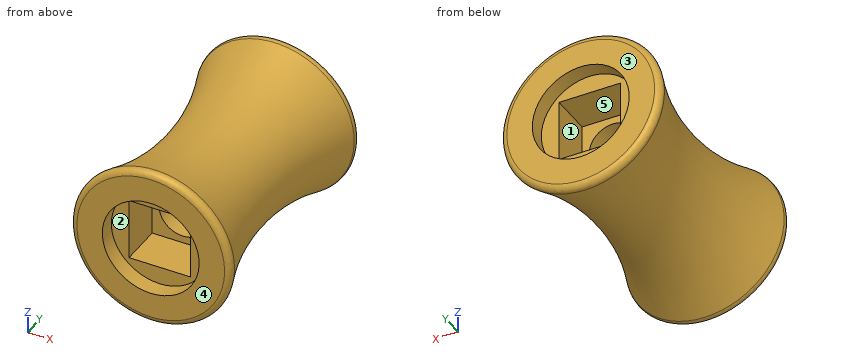
from build123d import *

# Parameters (mm, degrees)
SKETCH2_W           = 6.604
SKETCH2_H           = 6.604
CUT_EXTRUDE1_DEPTH  = 29.341210278
SKETCH3_R           = 5.207
CUT_EXTRUDE2_DEPTH  = 1.778
FILLET1_R           = 0.635
SKETCH4_W           = 6.604
SKETCH4_H           = 6.604
SKETCH4_R           = 2.54
BOSS_EXTRUDE1_DEPTH = 6.35


with BuildPart() as part:
    # Sketch1 → Revolve1 (revolve)
    with BuildSketch(Plane(origin=(0, 0, 0), x_dir=(0, 0, -1), z_dir=(1, 0, 0))):
        with BuildLine():
            Line((2.54, 0), (2.54, 25.4))
            Line((2.54, 25.4), (8.89, 25.4))
            ThreePointArc((8.89, 25.4), (6.239355663, 12.7), (8.89, 0))
            Line((8.89, 0), (2.54, 0))
        make_face()
    revolve(axis=Axis((0, 0, 0), (0, 1, 0)))

    # Sketch2 → Cut-Extrude1 (cut, through all)
    with BuildSketch(Plane.XZ):
        Rectangle(SKETCH2_W, SKETCH2_H)
    extrude(amount=-CUT_EXTRUDE1_DEPTH, mode=Mode.SUBTRACT)

    # Sketch3 → Cut-Extrude2 (cut)
    with BuildSketch(Plane.XZ):
        with Locations(Location((0, 0, 0), (0, 0, 270))):
            Circle(SKETCH3_R)
    cut_extrude2 = extrude(amount=-CUT_EXTRUDE2_DEPTH, mode=Mode.SUBTRACT)

    # Fillet1
    fillet1_edges = [part.edges().sort_by_distance(p)[0] for p in [
        (0, 25.4, 8.89),
        (0, 0, 8.89),
    ]]
    fillet(fillet1_edges, radius=FILLET1_R)

    # Mirror1: Cut-Extrude2 across plane
    add(cut_extrude2.mirror(Plane(origin=(0, 12.7, 0), x_dir=(0, 0, 1), z_dir=(0, -1, 0))), mode=Mode.SUBTRACT)

    # Sketch4 → Boss-Extrude1 (add, symmetric)
    with BuildSketch(Plane(origin=(0, 12.7, 0), x_dir=(-1, 0, 0), z_dir=(0, -1, 0))):
        Rectangle(SKETCH4_W, SKETCH4_H)
        with Locations(Location((0, 0, 0), (0, 0, 90))):
            Circle(SKETCH4_R, mode=Mode.SUBTRACT)
    extrude(amount=BOSS_EXTRUDE1_DEPTH, both=True)


solid = part.part
Can you work these out from the model? Positions are in its coordinate system, mm. Face numbers are marked on the shaded views. A direction names the side the tool comes from. Round coordinates to 2 decimals unless told otherwise and drop trailing zeros. Write each loop counter-clockwise with the first axis right and the second up, starting at its lowest first coordinate (ties: lowest second). Pieces come first, ordered by that corner, then holes. Notation, with made-up numbers: (16, 89) -> (25, 89) arc R21 ccw to (25, 125) -> close; hole circle Ø5 at (-21.5, -15). An arc over 180 degrees is marked (long way). Use one line per item in the form item = value. Start each with the question number.
Q1. Which directions (+Z, -Z, +X, -X, +Y, -Y) give clear straight access to the entire face, cutting with the end or side of a thin tool? Please do the marked faces 1, 2 and 3.
Q2. I'm going to push flat-ended pins straight in: P1, Ø1, axis at x = 2.5, z = -1, coming from the +Y side; P2, Ø1.4, axis at y = 22, z = 0, coming from the -X side; P3, Ø10, axis at x = -5.5, y = 18, coming from the -Z side; P4, Ø2, axis at x = 0.5, z = 0, coming from the -Y side. Where does each tip first touch, or does it pass through?
Q3. Imagine slicing it at B-B (y = 11.5). Please give me the cut outline in (x, z).
Q4. If I drill on probe 1 along X at (y, z) = (1.45, 0); probe 2 along Y at (x, z) = (-1.25, 4.75); probe 3 along Z at (x, y) = (-2.25, 3.5), over which ranges is the centre line in solid material (lowest first)? Write a range as [from, to].
Q5. Imagine slicing it at A-A (y = 3.5). Please give me the cut outline in (x, z).
Q6. We'd pull the mould along X, two halves only. Please class the marked faces 4 and 5: +X half, -X half, draft (parallel to the pull), parting line (faces both ways), or undercut.
Worked out:
q1.face_1 = +Y
q1.face_2 = -Y
q1.face_3 = +Z, -Z, +X, -X, +Y
q2.P1 = 19.05
q2.P2 = -7.86
q2.P3 = -7.23
q2.P4 = through
q3.outline = circle Ø12.52 at (0, 0); hole circle Ø5.08 at (0, 0)
q4.probe_1 = [-8.3, -5.21], [5.21, 8.3]
q4.probe_2 = [1.78, 23.62]
q4.probe_3 = [-7.26, -3.3], [3.3, 7.26]
q5.outline = circle Ø15.2 at (0, 0); hole (-3.3, -3.3) -> (3.3, -3.3) -> (3.3, 3.3) -> (-3.3, 3.3) -> close
q6.face_4 = draft
q6.face_5 = undercut
